The model under review builds one solid part; all positions refer to its coordinate system, in mm. A direction names the side the tool comes from. Give positions to 0.01 mm unless a question says otherwise; leave off trailing zeros. Loops run counter-clockwise (first coordinate to the right, second up) from the corner with the lowest first, then second, coordinate; pieces in that order, holes last. Notation, with made-up numbers: M 25.25,-28.75 L 56.25,-28.75 A10 cw 56.25,-21.75 Z; hole C 22.5,30.25 d10. An arc over 180 degrees is marked long. Return JSON: item names as keys, results as strings.
Autodesk Inventor part; units mm, degrees
ref_plane "YZ Plane" through (0, 0, 0) normal (1, 0, 0) x (0, 1, 0)
ref_plane "XZ Plane" through (0, 0, 0) normal (0, 1, 0) x (-1, 0, 0)
ref_plane "XY Plane" through (0, 0, 0) normal (0, 0, 1) x (1, 0, 0)
sketch "Sketch1" plane through (0, 0, 0) normal (0, 1, 0) x (-1, 0, 0)
  circle A0 centre (34.925, 5.5508) radius 13.97
  line L0 (69.85, 28.9263) -> (69.85, -106.7248)
  line L1 (0, -91.6029) -> (0, 13.8044)
  line L2 (-4.1782, 19.7715) -> (-65.6375, 42.1409)
  line L3 (-4.1782, -97.57) -> (-65.6375, -119.9394)
  line L4 (65.6718, 34.8933) -> (-52.6066, 77.9431)
  line L5 (65.6718, -112.6918) -> (-52.6066, -155.7416)
  line L6 (-69.4327, 50.2797) -> (-60.7454, 74.1479)
  line L7 (-69.4327, -128.0782) -> (-60.7454, -151.9464)
  arc A1 (-69.4327, 50.2797) -> (-65.6375, 42.1409) centre (-63.4657, 48.1079) ccw
  arc A2 (-52.6066, 77.9431) -> (-60.7454, 74.1479) centre (-54.7784, 71.9761) ccw
  arc A3 (-65.6375, -119.9394) -> (-69.4327, -128.0782) centre (-63.4657, -125.9064) ccw
  arc A4 (-60.7454, -151.9464) -> (-52.6066, -155.7416) centre (-54.7784, -149.7746) ccw
  arc A5 (69.85, 28.9263) -> (65.6718, 34.8933) centre (63.5, 28.9263) ccw
  arc A6 (65.6718, -112.6918) -> (69.85, -106.7248) centre (63.5, -106.7248) ccw
  arc A7 (-4.1782, -97.57) -> (0, -91.6029) centre (-6.35, -91.6029) ccw
  arc A8 (0, 13.8044) -> (-4.1782, 19.7715) centre (-6.35, 13.8044) ccw
  line L8 (-51.7378, 80.33) -> (66.5406, 37.2802)
  arc A9 (72.39, 28.9263) -> (66.5406, 37.2802) centre (63.5, 28.9263) ccw
  line L9 (72.39, 28.9263) -> (72.39, -106.7248)
  arc A10 (66.5406, -115.0786) -> (72.39, -106.7248) centre (63.5, -106.7248) ccw
  line L10 (66.5406, -115.0786) -> (-51.7378, -158.1285)
  arc A11 (-63.1323, -152.8152) -> (-51.7378, -158.1285) centre (-54.7784, -149.7746) ccw
  line L11 (-63.1323, -152.8152) -> (-71.8196, -128.947)
  arc A12 (-66.5063, -117.5525) -> (-71.8196, -128.947) centre (-63.4657, -125.9064) ccw
  line L12 (-66.5063, -117.5525) -> (-5.0469, -95.1832)
  arc A13 (-5.0469, -95.1832) -> (-2.54, -91.6029) centre (-6.35, -91.6029) ccw
  line L13 (-2.54, -91.6029) -> (-2.54, 13.8044)
  arc A14 (-2.54, 13.8044) -> (-5.0469, 17.3847) centre (-6.35, 13.8044) ccw
  line L14 (-5.0469, 17.3847) -> (-66.5063, 39.754)
  arc A15 (-71.8196, 51.1485) -> (-66.5063, 39.754) centre (-63.4657, 48.1079) ccw
  line L15 (-71.8196, 51.1485) -> (-63.1323, 75.0167)
  arc A16 (-51.7378, 80.33) -> (-63.1323, 75.0167) centre (-54.7784, 71.9761) ccw
  point P0 (0, 0)
  point P1 (0, 0)
  point P2 (0, 18.2508)
  point P3 (0, -96.0492)
  point P4 (-71.6046, 44.3127)
  point P5 (-71.6046, -122.1112)
  point P6 (69.85, 33.3726)
  point P7 (-58.5736, 80.115)
  point P8 (69.85, -111.1711)
  point P9 (-58.5736, -157.9135)
  dimension "d0" = 27.94
  dimension "d1" = 114.3
  dimension "d2" = 76.2
  dimension "d3" = 110
  dimension "d4" = 76.2
  dimension "d5" = 110
  dimension "d6" = 38.1
  dimension "d7" = 38.1
  dimension "d8" = 34.925
  dimension "d9" = 12.7
  dimension "d10" = 6.35
  dimension "d11" = 6.35
  dimension "d12" = 69.85
  dimension "d13" = 2.54
extrude "Extrusion1" add sketch "Sketch1" along normal blind 36.83 contours L8 A9 L9 A10 L10 A11 L11 A12 L12 A13 L13 A14 L14 A15 L15 A16
sketch "Sketch4" plane through (0, 0, 0) normal (0, 1, 0) x (-1, 0, 0)
  arc A0 (65.6718, -112.6918) -> (69.85, -106.7248) centre (63.5, -106.7248) ccw
  line L0 (-4.1782, -97.57) -> (-65.6375, -119.9394)
  line L1 (65.6718, -112.6918) -> (-52.6066, -155.7416)
  arc A1 (-4.1782, -97.57) -> (0, -91.6029) centre (-6.35, -91.6029) ccw
  line L2 (-4.1782, 19.7715) -> (-65.6375, 42.1409)
  arc A2 (-65.6375, -119.9394) -> (-69.4327, -128.0782) centre (-63.4657, -125.9064) ccw
  line L3 (-69.4327, -128.0782) -> (-60.7454, -151.9464)
  arc A3 (-60.7454, -151.9464) -> (-52.6066, -155.7416) centre (-54.7784, -149.7746) ccw
  line L4 (0, -91.6029) -> (0, 13.8044)
  line L5 (69.85, 28.9263) -> (69.85, -106.7248)
  arc A4 (0, 13.8044) -> (-4.1782, 19.7715) centre (-6.35, 13.8044) ccw
  arc A5 (69.85, 28.9263) -> (65.6718, 34.8933) centre (63.5, 28.9263) ccw
  line L6 (65.6718, 34.8933) -> (-52.6066, 77.9431)
  line L7 (-69.4327, 50.2797) -> (-60.7454, 74.1479)
  arc A6 (-52.6066, 77.9431) -> (-60.7454, 74.1479) centre (-54.7784, 71.9761) ccw
  arc A7 (-69.4327, 50.2797) -> (-65.6375, 42.1409) centre (-63.4657, 48.1079) ccw
  line L8 (-51.7378, 80.33) -> (66.5406, 37.2802)
  arc A8 (72.39, 28.9263) -> (66.5406, 37.2802) centre (63.5, 28.9263) ccw
  line L9 (72.39, 28.9263) -> (72.39, -106.7248)
  arc A9 (66.5406, -115.0786) -> (72.39, -106.7248) centre (63.5, -106.7248) ccw
  line L10 (66.5406, -115.0786) -> (-51.7378, -158.1285)
  arc A10 (-63.1323, -152.8152) -> (-51.7378, -158.1285) centre (-54.7784, -149.7746) ccw
  line L11 (-63.1323, -152.8152) -> (-71.8196, -128.947)
  arc A11 (-66.5063, -117.5525) -> (-71.8196, -128.947) centre (-63.4657, -125.9064) ccw
  line L12 (-66.5063, -117.5525) -> (-5.0469, -95.1832)
  arc A12 (-5.0469, -95.1832) -> (-2.54, -91.6029) centre (-6.35, -91.6029) ccw
  line L13 (-2.54, -91.6029) -> (-2.54, 13.8044)
  arc A13 (-2.54, 13.8044) -> (-5.0469, 17.3847) centre (-6.35, 13.8044) ccw
  line L14 (-5.0469, 17.3847) -> (-66.5063, 39.754)
  arc A14 (-71.8196, 51.1485) -> (-66.5063, 39.754) centre (-63.4657, 48.1079) ccw
  line L15 (-71.8196, 51.1485) -> (-63.1323, 75.0167)
  arc A15 (-51.7378, 80.33) -> (-63.1323, 75.0167) centre (-54.7784, 71.9761) ccw
  point P0 (0, 0)
  point P1 (0, 0)
  point P2 (0, -96.0492)
  point P3 (69.85, -111.1711)
  point P4 (-71.6046, -122.1112)
  point P5 (-58.5736, -157.9135)
  point P6 (0, 18.2508)
  point P7 (-71.6046, 44.3127)
  point P8 (69.85, 33.3726)
  point P9 (-58.5736, 80.115)
  point P10 (0, 0)
  dimension "d17" = 114.3
  dimension "d18" = 76.2
  dimension "d19" = 110
  dimension "d20" = 76.2
  dimension "d21" = 110
  dimension "d22" = 38.1
  dimension "d23" = 38.1
  dimension "d26" = 6.35
  dimension "d27" = 6.35
  dimension "d28" = 69.85
  dimension "d29" = 2.54
extrude "Extrusion2" add sketch "Sketch4" along normal blind 2.54 contours L1 A3 L3 A2 L0 A1 L4 A4 L2 A7 L7 A6 L6 A5 L5 A0
properties part number "CONTROLLER CASE"
1) Consider section C-C on z = -41.5. Write out the cut boundary in (x, y), then the cut area to 3 significant figures.
From the geometry:
{"outline": "M -72.39,0 L 2.54,0 L 2.54,36.83 L 0,36.83 L 0,2.54 L -69.85,2.54 L -69.85,36.83 L -72.39,36.83 Z", "area": "365 mm²"}
2) Insertion check: pin 1 (10 mm diameter, centred on x = -42, z = 25, fed in from -Y); pin 2 (10 mm diameter, centred on x = 41, y = 32.5, fed in from -Z); pin 3 (10.5 mm diameter, centred on y = 16.5, z = -25.5, fed in from +X); pin 4 (3 mm diameter, centred on x = 24.5, y = 29, fed in from +Z). Each pin has a flat end and moves straight along its axis. Give the tip position at first contact, or say it passes through.
From the geometry:
{"pin 1": "y = 0", "pin 2": "z = -156.04", "pin 3": "x = 2.54", "pin 4": "z = 70.96"}
3) Consider section B-B on x = 42.5. Write out the cut boundary in (y, z), then the cut area to 3 significant figures.
From the geometry:
{"outline": "M 0,-154.77 L 36.83,-154.77 L 36.83,-152.06 L 2.54,-152.06 L 2.54,-111.52 L 36.83,-111.52 L 36.83,-108.81 L 0,-108.81 Z; M 0,31.02 L 36.83,31.02 L 36.83,33.72 L 2.54,33.72 L 2.54,74.26 L 36.83,74.26 L 36.83,76.97 L 0,76.97 Z", "area": "604 mm²"}
4) Tool access review of faces 1 (the face through (-15, 0, -37)), 2 (the face through (1.18, 19.44, 17.49)), 3 (the face through (2.54, 18, -40)): name each direction out of +Z, -Z, +X, -X, +Y, -Y from which nothing blocks a thin tool from reaching the whole face with its end or side.
From the geometry:
{"face 1": "+Z, -Z, +X, -X, -Y", "face 2": "+Y", "face 3": "+X, +Y, -Y"}
5) Wall thickness on L1, parallel to X at y = 8, z = -90; L2, parallel to Z at x = 2, y = 3.5; L3, parallel to Z at x = 28.5, y = 19.5: over which ranges is each line inside the solid? List them lowest first. Write a range as from..to.
From the geometry:
{"L1": "-72.39..-69.85, 0..2.54", "L2": "-140.03..-137.32, -96.23..18.43, 59.52..62.23", "L3": "-149.67..-146.97, -106.42..-103.72, 25.92..28.62, 69.17..71.87"}
6) Consider section D-D on x = -16. Write out the cut boundary in (y, z), then the cut area to 3 significant figures.
From the geometry:
{"outline": "M 0,-133.47 L 36.83,-133.47 L 36.83,-130.77 L 2.54,-130.77 L 2.54,52.97 L 36.83,52.97 L 36.83,55.68 L 0,55.68 Z", "area": "666 mm²"}
7) The part is to be moulded in two halves that separate along X. For faces 4 (the face through (36.207, 18.157, -106.524)), 5 (the face through (1.117, 19.445, -95.201)), 6 (the face through (-68.67, 19.44, 32.61)), 7 (the face through (-70.738, 18.157, 34.087)), say which applies: released by +X, released by -X, zero draft, split by the parting line, or undercut.
From the geometry:
{"face 4": "released by +X", "face 5": "undercut", "face 6": "undercut", "face 7": "released by -X"}
